Geometry check sheet. Reference: the model listing, model coordinates, mm. A direction names the side the tool comes from. Coordinates: 2 decimals unless noted, no trailing zeros. Write each loop counter-clockwise with the first axis right and the second up, starting at its lowest first coordinate (ties: lowest second). Pieces come first, ordered by that corner, then holes. Notation, with made-up numbers: (-35, 71.5) -> (-23, 71.5) arc R22 ccw to (-23, 98.5) -> close; hole circle Ø4 at (-31, 21). An arc over 180 degrees is marked (long way). Answer as CSV lines item,"result".
```python
from build123d import *

# Parameters (mm, degrees)
F0_R     = 25
F1_DEPTH = 665.8
F2_R     = 25
F2_R_2   = 17.5
F3_DEPTH = 97
F4_R     = 25
F4_R_2   = 17.5
F5_DEPTH = 17
F7_DEPTH = 67


with BuildPart() as f1:
    # F0 (on Front) → F1 (new body)
    with BuildSketch(Plane.XZ):
        with Locations((-99.979594, 13.985418)):
            Circle(F0_R)
    extrude(amount=F1_DEPTH)

    # F2 (on face) → F3 (cut)
    with BuildSketch(Plane.XZ.offset(665.8)):
        with Locations((-99.979594, 13.985418)):
            Circle(F2_R)
        with Locations((-99.979594, 13.985418)):
            Circle(F2_R_2, mode=Mode.SUBTRACT)
    extrude(amount=-F3_DEPTH, mode=Mode.SUBTRACT)

    # F4 (on face) → F5 (cut)
    with BuildSketch(Plane.XZ):
        with Locations((-99.979594, 13.985418)):
            Circle(F4_R)
        with Locations((-99.905901, 14.123433)):
            Circle(F4_R_2, mode=Mode.SUBTRACT)
    extrude(amount=F5_DEPTH, mode=Mode.SUBTRACT)

    # F6 (on face) → F7 (cut)
    with BuildSketch(Plane.XZ.offset(665.8)):
        with BuildLine():
            Line((-104.960215, 30.756418), (-104.960215, 26.485418))
            Line((-104.960215, 26.485418), (-94.960215, 26.485418))
            Line((-94.960215, 26.485418), (-94.960215, 30.750138))
            ThreePointArc((-94.960215, 30.750138), (-99.910954, 31.485283), (-104.867307, 30.788997))
            ThreePointArc((-104.867307, 30.788997), (-104.913788, 30.772784), (-104.960215, 30.756418))
        make_face()
    extrude(amount=-F7_DEPTH, mode=Mode.SUBTRACT)


solid = f1.part
```
Item 1: Cross-section at C-C, the plane y = -392. Record the cut outline in (x, z), plus the area to 3 significant figures.
Responses:
outline,"circle Ø50 at (-99.98, 13.99)"
area,"1,960 mm2"
Item 2: Depth check by flat-ended pin: pin 1 Ø3 at (y, z) = (-87.5, 19) entering from -X; pin 2 Ø8 at (x, z) = (-87, 31) entering from +Y; pin 3 Ø5 at (x, y) = (-107.5, -489) entering from +Z; pin 4 Ø6 at (x, y) = (-104.5, -364.5) entering from -Z. Enter the tip coordinate at first touch or a pass-through.
Responses:
pin 1,"stops at x = -124.73"
pin 2,"stops at y = 0"
pin 3,"stops at z = 38.48"
pin 4,"stops at z = -10.97"
Item 3: Cross-section at B-B, the plane x = -88. Record the cut outline in (y, z), plus the area to 3 significant figures.
Responses:
outline,"(-665.8, 1.23) -> (-568.8, 1.23) -> (-568.8, -7.96) -> (-17, -7.96) -> (-17, 1.3) -> (0, 1.3) -> (0, 26.95) -> (-17, 26.95) -> (-17, 35.93) -> (-568.8, 35.93) -> (-568.8, 26.74) -> (-665.8, 26.74) -> close"
area,"27,100 mm2"
Item 4: Set-up check for faces 1 (the cylindrical face through (-90.5, -8.38, 28.88)), 2 (the flat face through (-100, -665.8, 14)), 3 (the flat face through (-95, -568.8, 31)): record each of +Z, -Z, +X, -X, +Y, -Y from which the full face is reachable in a straight line by a thin tool's end or side.
Responses:
face 1,"+Y"
face 2,"+Z, -Z, +X, -X, -Y"
face 3,"-Y"
Item 5: Thickness scan on probe 1 along Y at (x, z) = (-110.5, 33); probe 2 along X at (y, z) = (-229, 13); probe 3 along Z at (x, y) = (-103, -166). Record the ranges inside material, lowest first.
Responses:
probe 1,"y = -568.8 to -17"
probe 2,"x = -124.96 to -75"
probe 3,"z = -10.83 to 38.8"
Item 6: Cross-section at D-D, the plane y = -588. Record the cut outline in (x, z).
Responses:
outline,"circle Ø35 at (-99.98, 13.99)"
Item 7: Cross-section at A-A, the plane z = 8.5. Record the cut outline in (x, y), plus the area to 3 significant figures.
Responses:
outline,"(-124.37, -568.8) -> (-116.6, -568.8) -> (-116.6, -665.8) -> (-83.36, -665.8) -> (-83.36, -568.8) -> (-75.59, -568.8) -> (-75.59, -17) -> (-83.33, -17) -> (-83.33, 0) -> (-116.48, 0) -> (-116.48, -17) -> (-124.37, -17) -> close"
area,"30,700 mm2"
